from build123d import *

# Parameters (mm, degrees)
BLANKSKE_W        = 25
BLANKSKE_H        = 5.5
BLANK_DEPTH       = 7.7
TOOTHCUTSIM_DEPTH = 27.730881018
TEETHCUTS_COUNT   = 17
TEETHCUTS_PITCH   = 1.570796325


with BuildPart() as part:
    # BlankSke → Blank (new body)
    with BuildSketch(Plane.XY):
        with Locations((12.5, 2.75)):
            Rectangle(BLANKSKE_W, BLANKSKE_H)
    extrude(amount=-BLANK_DEPTH)

    # TooCutSkeSim → ToothCutSim (cut, through all)
    with BuildSketch(Plane.XY):
        Polygon((0.222217685, 4.375), (-0.222217685, 4.375), (-0.640929042, 5.5254), (0.640929042, 5.5254), align=None)
    toothcutsim = extrude(amount=-TOOTHCUTSIM_DEPTH, mode=Mode.SUBTRACT)

    # TeethCuts: ToothCutSim ×17
    with Locations(*[(i * TEETHCUTS_PITCH, 0, 0) for i in range(1, TEETHCUTS_COUNT)]):
        add(toothcutsim, mode=Mode.SUBTRACT)


solid = part.part
Read the model definition and answer for the solid it produces. Units are mm, in the model's axes. A direction names the side the tool comes from. Round coordinates to 2 decimals unless told otherwise and drop trailing zeros. Use a Markdown table: item, result.
1) For a pull along X with two mould halves and no side action, classify faces 1 (the flat face through (12, 0, -4)), 2 (the flat face through (25, 2, -4)), 3 (the flat face through (20.85, 4.95, -3.8)) as pulls with the +X half, pulls with the -X half, needs draft (parallel to the pull), parting line crosses it, or undercut.
Answers follow:
| item | result |
|---|---|
| face 1 | needs draft |
| face 2 | pulls with the +X half |
| face 3 | undercut |
2) A tool of negligible diameter and unlimited length cuts with its end or side. For faces 4 (the flat face through (12, 2, 0)), 5 (the flat face through (10.57, 4.93, -3.8)), from which of +Z, -Z, +X, -X, +Y, -Y can it reach the whole face along a straight path? Write none if from no direction.
Answers follow:
| item | result |
|---|---|
| face 4 | +Z, +X, -X, +Y, -Y |
| face 5 | +Z, -Z, +Y |
3) The part is cut by section A-A (y = 4.65). Give the number of separate pieces and of enclosed holes in the cut face, plus the area to 3 significant figures.
Answers follow:
| item | result |
|---|---|
| separate pieces | 16 |
| enclosed holes | 0 |
| area | 114 mm2 |
4) A straight line is drawn through the part: line 1 along Y through (x, z) = (17.25, -2) (3 decimals). Find the intervals that lie inside material, in ascending order. Write a range as [from, to].
Answers follow:
| item | result |
|---|---|
| line 1 | y = [0, 4.375] |
